from build123d import *

# Parameters (mm, degrees)
SKETCH1_R          = 16.5354
EXTRUDE1_DEPTH     = 49.7332
CUT_EXTRUDE1_DEPTH = 19.84248
SKETCH12_W         = 4.6736
SKETCH12_H         = 1.5113
SKETCH13_W         = 7.2644
SKETCH13_H         = 10.3251
S2D0011_W          = 4.0132
S2D0011_H          = 9.652
CIRPATTERN2_COUNT  = 6


with BuildPart() as part:
    # Sketch1 → Extrude1 (new body)
    with BuildSketch(Plane.XY):
        Circle(SKETCH1_R)
    extrude(amount=EXTRUDE1_DEPTH)

    # Sketch2 → Cut-Extrude1 (cut, symmetric)
    with BuildSketch(Plane(origin=(0, 0, 0), x_dir=(0, 0, 1), z_dir=(1, 0, 0))):
        with BuildLine():
            Line((42.8752, 16.5354), (42.8752, 14.76375))
            ThreePointArc((42.8752, 14.76375), (43.023989755, 14.404539755), (43.3832, 14.25575))
            Line((43.3832, 14.25575), (49.7332, 14.25575))
            Line((49.7332, 14.25575), (49.7332, 16.5354))
            Line((49.7332, 16.5354), (42.8752, 16.5354))
        make_face()
    cut_extrude1 = extrude(amount=CUT_EXTRUDE1_DEPTH, both=True, mode=Mode.SUBTRACT)

    # Sketch10 → Cut-Revolve1 (revolve, cut)
    with BuildSketch(Plane(origin=(0, 0, 0), x_dir=(0, 0, -1), z_dir=(1, 0, 0)), mode=Mode.PRIVATE) as cut_revolve1_sk:
        Polygon((-49.7332, 15.494), (-43.3832, 15.494), (-42.3418, 16.5354), (-49.7332, 16.5354), align=None)
    revolve(cut_revolve1_sk.sketch.rotate(Axis((0, 0, 50.10277), (0, 0, -1)), 90), axis=Axis((0, 0, 50.10277), (0, 0, -1)), mode=Mode.SUBTRACT)  # turned: the seam where the file's is

    # Sketch11 → Cut-Revolve2 (revolve, cut)
    with BuildSketch(Plane(origin=(0, 0, 0), x_dir=(0, 0, 1), z_dir=(1, 0, 0)), mode=Mode.PRIVATE) as cut_revolve2_sk:
        Polygon((0, 15.5067), (8.2804, 15.5067), (9.3091, 16.5354), (0, 16.5354), align=None)
    revolve(cut_revolve2_sk.sketch.rotate(Axis((0, 0, -0.465455), (0, 0, 1)), 270), axis=Axis((0, 0, -0.465455), (0, 0, 1)), mode=Mode.SUBTRACT)  # turned: the seam where the file's is

    # Sketch12 → Cut-Revolve3 (revolve, cut)
    with BuildSketch(Plane(origin=(0, 0, 0), x_dir=(0, 0, -1), z_dir=(1, 0, 0)), mode=Mode.PRIVATE) as cut_revolve3_sk:
        with Locations((-2.3368, 14.75105)):
            Rectangle(SKETCH12_W, SKETCH12_H)
    revolve(cut_revolve3_sk.sketch.rotate(Axis((0, 0, 4.90728), (0, 0, -1)), 270), axis=Axis((0, 0, 4.90728), (0, 0, -1)), mode=Mode.SUBTRACT)  # turned: the seam where the file's is

    # Sketch13 → Revolve1 (revolve)
    with BuildSketch(Plane(origin=(0, 0, 0), x_dir=(0, 0, -1), z_dir=(1, 0, 0)), mode=Mode.PRIVATE) as revolve1_sk:
        with Locations((-53.3654, 5.16255)):
            Rectangle(SKETCH13_W, SKETCH13_H)
    revolve(revolve1_sk.sketch.rotate(Axis((0, 0, 57.36082), (0, 0, -1)), 270), axis=Axis((0, 0, 57.36082), (0, 0, -1)))  # turned: the seam where the file's is

    # S2D0011 → Cut-Revolve4 (revolve, cut)
    with BuildSketch(Plane(origin=(-4.0132, 0, 56.9976), x_dir=(-1, 0, 0), z_dir=(0, 1, 0))):
        with Locations((-2.0066, -4.826)):
            Rectangle(S2D0011_W, S2D0011_H)
    revolve(axis=Axis((0, 0, 32.002650052), (0, 0, 1)), mode=Mode.SUBTRACT)

    # Sketch15 → Cut-Revolve5 (revolve, cut)
    with BuildSketch(Plane(origin=(0, 0, 0), x_dir=(0, 0, -1), z_dir=(1, 0, 0)), mode=Mode.PRIVATE) as cut_revolve5_sk:
        with BuildLine():
            Line((-56.9976, 8.7376), (-56.142107199, 9.97462236))
            ThreePointArc((-56.142107199, 9.97462236), (-55.851004442, 10.232167854), (-55.4736, 10.3251))
            Line((-55.4736, 10.3251), (-56.9976, 10.3251))
            Line((-56.9976, 10.3251), (-56.9976, 8.7376))
        make_face()
    revolve(cut_revolve5_sk.sketch.rotate(Axis((0, 0, 57.0738), (0, 0, -1)), 270), axis=Axis((0, 0, 57.0738), (0, 0, -1)), mode=Mode.SUBTRACT)  # turned: the seam where the file's is

    # CirPattern2: Cut-Extrude1 ×6 about axis
    cirpattern2_axis = Axis((0, 0, 0), (0, 0, 1))
    for i in range(1, CIRPATTERN2_COUNT):
        add(cut_extrude1.rotate(cirpattern2_axis, i * 360 / CIRPATTERN2_COUNT), mode=Mode.SUBTRACT)


solid = part.part
Can you work these out from the model? Positions are in its coordinate system, mm. A direction names the side the tool comes from. Coordinates: 2 decimals unless noted, no trailing zeros. Write each loop counter-clockwise with the first axis right and the second up, starting at its lowest first coordinate (ties: lowest second). Pieces come first, ordered by that corner, then holes. Notation, with made-up numbers: (-30, 11) -> (0, 11) arc R5 cw to (0, 18) -> close; hole circle Ø1 at (2, 62.5). An arc over 180 degrees is marked (long way). Answer as CSV lines item,"result".
1) Will these pins go through, and if not, where does the flat tip stop? P1, Ø1.9, axis at x = -11.5, y = 9, coming from the +Z side; P2, Ø12, axis at x = 9, z = 33.5, coming from the +Y side; P3, Ø1.5, axis at y = 8, z = 26.5, coming from the -X side.
Check result:
P1,"z = 49.73"
P2,"y = 16.26"
P3,"x = -14.86"
2) If we section it at C-C on z = 25.5: Please give me the cut outline in (x, y).
Check result:
outline,"circle Ø33.07 at (0, 0)"
3) If I drill on line 1 (Y direction, x = 0, z = 52.75); line 2 (Z direction, x = -2.5, y = -3); line 3 (Z direction, x = 13, y = 7.5), over which ranges is the centre line in solid material (lowest first)? Write a range as from..to.
Check result:
line 1,"-10.33..-4.01, 4.01..10.33"
line 2,"0..47.35"
line 3,"4.67..42.88"
4) If we mould it in two halves opening along Y, with no side actions, what happens to faces 5 (the flat face through (0, 0, 47.346)), 6 (the flat face through (-12.303, -7.201, 46.514)), 7 (the cylindrical face through (7.724, 13.431, 46.514)), 8 (the cylindrical face through (-15.494, -0.026, 46.514))? For each: +Y half, -Y half, draft (parallel to the pull), parting line (faces both ways), or undercut.
Check result:
face 5,"undercut"
face 6,"-Y half"
face 7,"+Y half"
face 8,"parting line"
5) On a 3-axis mill with a long thin cutter (end or side, diameter ignored), from which of +Z, -Z, +X, -X, +Y, -Y can I reach the whole of each face in a straight line? I mean faces 1 (the cylindrical face through (-7.77, 13.405, 46.514)), 2 (the cylindrical face through (11.106, -8.516, 2.304)), 3 (the cylindrical face through (-9.54, -3.95, 52.56)), 4 (the flat face through (12.39, -7.05, 46.51)). Say none if no direction works.
Check result:
face 1,"+Z, -X, +Y"
face 2,"-Z"
face 3,"+Z"
face 4,"+Z, +X, -Y"
6) If we section it at A-A on y = 0: Please give me the cut outline in (x, z).
Check result:
outline,"(-16.54, 9.31) -> (-15.51, 8.28) -> (-15.51, 4.67) -> (-14, 4.67) -> (-14, 0) -> (14, 0) -> (14, 4.67) -> (15.51, 4.67) -> (15.51, 8.28) -> (16.54, 9.31) -> (16.54, 42.34) -> (15.49, 43.38) -> (15.49, 49.73) -> (10.33, 49.73) -> (10.33, 55.47) arc R0.81 ccw to (9.97, 56.14) -> (8.74, 57) -> (4.01, 57) -> (4.01, 47.35) -> (-4.01, 47.35) -> (-4.01, 57) -> (-8.74, 57) -> (-9.97, 56.14) arc R0.81 ccw to (-10.33, 55.47) -> (-10.33, 49.73) -> (-15.49, 49.73) -> (-15.49, 43.38) -> (-16.54, 42.34) -> close"
